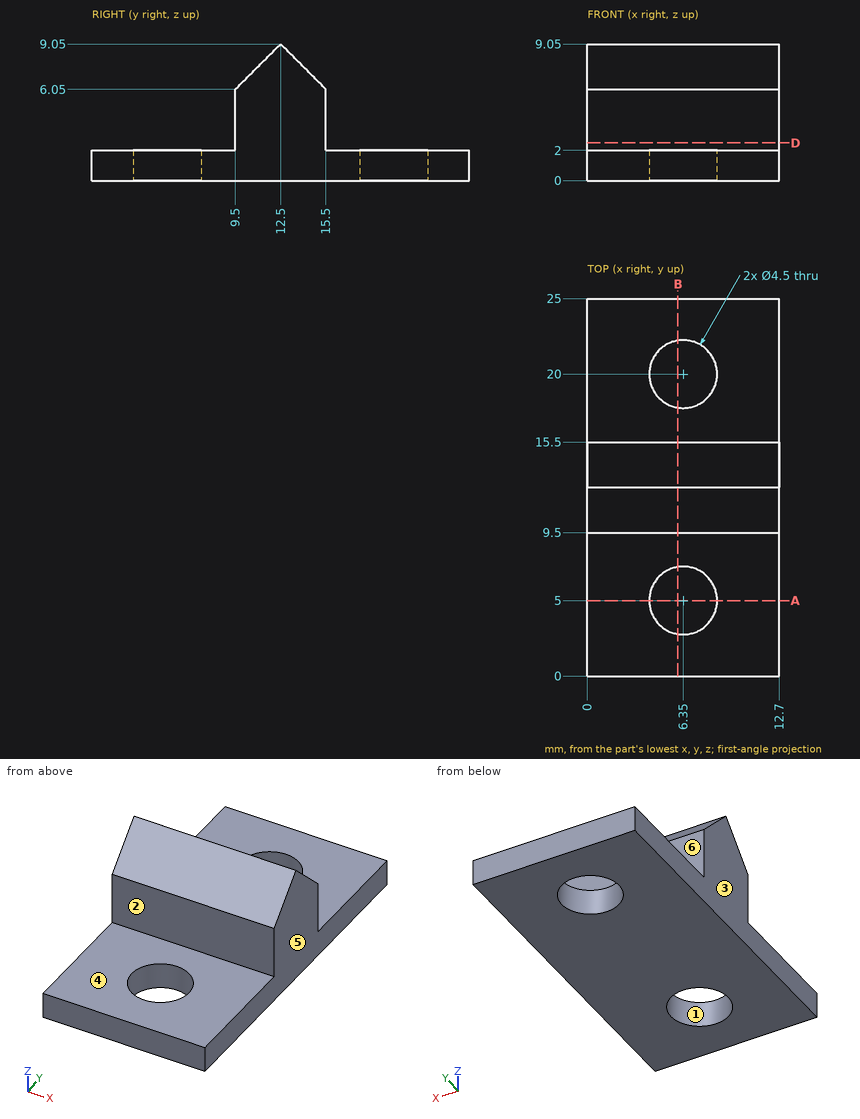
Job drawing, mm, ordinate dimensions from the low corner. One solid piece. A direction names the side the tool comes from. Round coordinates to 2 decimals unless told otherwise and drop trailing zeros. Loops run counter-clockwise (first coordinate to the right, second up) from the corner with the lowest first, then second, coordinate; pieces in that order, holes last. Notation, with made-up numbers: (26, 1) -> (57, 1) arc R15 ccw to (57, 14) -> close; hole circle Ø3 at (59.25, 51.5). An arc over 180 degrees is marked (long way). One line per item, written item: value. Start each with the question number.
Q1. 3-axis set-ups, long thin cutter, end or side, ignore diameter. For the marked faces 4, 5 and 6: which of +Z, -Z, +X, -X, +Y, -Y reach the whole face in a straight line?
Q2. Two-plate mould, pull along X, no slides. Class the marked faces 1, 2 and 3: released by +X, released by -X, zero draft, split by the parting line, or undercut.
Q3. Cut at B-B on x = 6. Count the separate pieces of the cut face and the enclosed holes in it, plus the area to 3 significant figures.
Q4. Cut at D-D on z = 2.5. List the corners of the cut face in (x, y), plus the area to 3 significant figures.
Q5. Drop flat-ended pins along their axis: pin 1 Ø3.5 at (x, y) = (6.35, 20) entering from -Z; pin 2 Ø5 at (x, z) = (9, 5) entering from -Y; pin 3 Ø1.5 at (y, z) = (16, 3.5) entering from -X; pin 4 Ø7 at (x, y) = (6.35, 5) entering from +Z. Give the stop position or say it passes through.
Q6. Probe line 1 along Y through (x, z) = (6.35, 0.8); line 2 along Z through (x, y) = (11, 18.75); line 3 along Y through (x, z) = (5.25, 4). List the from-to ranges inside material, lowest first.
Q7. Cut at A-A on y = 5. List the corners of the cut face in (x, z).
Computed:
1. face 4: +Z, +X, -X, -Y
1. face 5: +Z, -Z, +X, +Y, -Y
1. face 6: +Z, +X, -X, +Y
2. face 1: undercut
2. face 2: zero draft
2. face 3: released by -X
3. separate pieces: 3
3. enclosed holes: 0
3. area: 65.5 mm²
4. outline: (0, 9.5) -> (12.7, 9.5) -> (12.7, 15.5) -> (0, 15.5) -> close
4. area: 76.2 mm²
5. pin 1: through
5. pin 2: y = 9.5
5. pin 3: x = 0
5. pin 4: z = 2
6. line 1: 0 to 2.75, 7.25 to 17.75, 22.25 to 25
6. line 2: 0 to 2
6. line 3: 9.5 to 15.5
7. outline: (0, 0) -> (4.1, 0) -> (4.1, 2) -> (0, 2) -> close; (8.6, 0) -> (12.7, 0) -> (12.7, 2) -> (8.6, 2) -> close
